Design review of the part built by this model. Coordinates are the model's own, in mm. A direction names the side the tool comes from. Round coordinates to 2 decimals unless told otherwise and drop trailing zeros. Order: outer loops, then holes, each group sorted by start corner. A loop starts at its lowest first (then second) coordinate and runs counter-clockwise, first axis right, second up.
from build123d import *

# Parameters (mm, degrees)
CUT_EXTRUDE_2_REACH      = 9.602
PATTERN_CIRCULAR_3_COUNT = 11
SKETCH_7_R               = 3.7
EXTRUDE_1_DEPTH          = 0.5
SKETCH_8_R               = 1.75
CUT_EXTRUDE_3_DEPTH      = 0.25
EXTRUDE_START            = 0.5
SKETCH_9_R               = 3.7
EXTRUDE_2_DEPTH          = 0.5
SKETCH_11_R              = 1.55
CUT_EXTRUDE_5_DEPTH      = 3
SKETCH_13_R              = 0.5625
CUT_EXTRUDE_7_DEPTH      = 9.739565207


with BuildPart() as part:
    # Sketch 1 → Revolve 1 (revolve)
    with BuildSketch(Plane.XY, mode=Mode.PRIVATE) as revolve_1_sk:
        Polygon((0, 1), (0, 3.301), (6, 3.301), (6, 2.2264), (6, 1), align=None)
    revolve(revolve_1_sk.sketch.rotate(Axis((0, 0, 0), (1, 0, 0)), 90), axis=Axis((0, 0, 0), (1, 0, 0)))

    # Sketch 6 → Cut-Extrude 2 (cut, up to next)
    with BuildSketch(Plane(origin=(0, 0, 0), x_dir=(0, 0, -1), z_dir=(1, 0, 0)), mode=Mode.PRIVATE) as cut_extrude_2_sk1:
        with BuildLine():
            Line((0.620299767, 3.127317535), (0.514085384, 2.835495915))
            ThreePointArc((0.514085384, 2.835495915), (0.376876254, 2.662359121), (0.163302545, 2.605888194))
            ThreePointArc((0.163302545, 2.605888194), (0, 2.611), (-0.163302545, 2.605888194))
            ThreePointArc((-0.163302545, 2.605888194), (-0.376876254, 2.662359121), (-0.514085384, 2.835495915))
            Line((-0.514085384, 2.835495915), (-0.620299767, 3.127317535))
            ThreePointArc((-0.620299767, 3.127317535), (-0.680969197, 3.197392704), (-0.772898084, 3.209241273))
            ThreePointArc((-0.772898084, 3.209241273), (-0.835941408, 3.193399906), (-0.898660577, 3.176320224))
            Line((-0.898660577, 3.176320224), (-1.396756451, 4.544827391))
            ThreePointArc((-1.396756451, 4.544827391), (0, 4.754617188), (1.396756451, 4.544827391))
            Line((1.396756451, 4.544827391), (0.898660577, 3.176320224))
            ThreePointArc((0.898660577, 3.176320224), (0.835941408, 3.193399906), (0.772898084, 3.209241273))
            ThreePointArc((0.772898084, 3.209241273), (0.680969197, 3.197392704), (0.620299767, 3.127317535))
        make_face()
    cut_extrude_2_tool1 = extrude(cut_extrude_2_sk1.sketch, amount=CUT_EXTRUDE_2_REACH, mode=Mode.PRIVATE) & part.part
    cut_extrude_2 = cut_extrude_2_tool1.solids().sort_by_distance((0, 3.839085, 0))[0]
    add(cut_extrude_2, mode=Mode.SUBTRACT)

    # Pattern Circular 3: Cut-Extrude 2 ×11 about axis
    pattern_circular_3_axis = Axis((0, 0, 0), (1, 0, 0))
    for i in range(1, PATTERN_CIRCULAR_3_COUNT):
        add(cut_extrude_2.rotate(pattern_circular_3_axis, i * 360 / PATTERN_CIRCULAR_3_COUNT), mode=Mode.SUBTRACT)

    # Sketch 7 → Extrude 1 (add)
    with BuildSketch(Plane.ZY):
        Circle(SKETCH_7_R)
    extrude(amount=EXTRUDE_1_DEPTH)

    # Sketch 8 → Cut-Extrude 3 (cut)
    with BuildSketch(Plane.ZY.offset(0.5)):
        Circle(SKETCH_8_R)
    extrude(amount=-CUT_EXTRUDE_3_DEPTH, mode=Mode.SUBTRACT)

    # Sketch 9 → Extrude 2 (add)
    with BuildSketch(Plane(origin=(6, 0, 0), x_dir=(0, 0, -1), z_dir=(1, 0, 0)).offset(EXTRUDE_START)):
        with Locations(Location((0, 0, 0), (0, 0, 180))):
            Circle(SKETCH_9_R)
    extrude(amount=-EXTRUDE_2_DEPTH)

    # Sketch 11 → Cut-Extrude 5 (cut)
    with BuildSketch(Plane.ZY.offset(0.25)):
        Circle(SKETCH_11_R)
    extrude(amount=-CUT_EXTRUDE_5_DEPTH, mode=Mode.SUBTRACT)

    # Sketch 13 → Cut-Extrude 7 (cut, through all)
    with BuildSketch(Plane(origin=(6.5, 0, 0), x_dir=(0, 0, -1), z_dir=(1, 0, 0))):
        Circle(SKETCH_13_R)
    extrude(amount=-CUT_EXTRUDE_7_DEPTH, mode=Mode.SUBTRACT)


solid = part.part
1) Take a section at A-A on z = 0. Give the boundary of the cut face in (x, y), plus the area to 3 significant figures.
Results:
outline: (-0.5, -3.7) - (0, -3.7) - (0, -3.3) - (6, -3.3) - (6, -3.7) - (6.5, -3.7) - (6.5, -0.56) - (6, -0.56) - (6, -1) - (2.75, -1) - (2.75, -1.55) - (-0.25, -1.55) - (-0.25, -1.75) - (-0.5, -1.75) - close; (-0.5, 1.75) - (-0.25, 1.75) - (-0.25, 1.55) - (2.75, 1.55) - (2.75, 1) - (6, 1) - (6, 0.56) - (6.5, 0.56) - (6.5, 3.7) - (6, 3.7) - (6, 2.61) - (0, 2.61) - (0, 3.7) - (-0.5, 3.7) - close
area: 25.6 mm2
2) Take a section at B-B on y = 0. Give the boundary of the cut face in (x, z), plus the area to 3 significant figures.
Results:
outline: (-0.5, -3.7) - (0, -3.7) - (0, -2.69) - (6, -2.69) - (6, -3.7) - (6.5, -3.7) - (6.5, -0.56) - (6, -0.56) - (6, -1) - (2.75, -1) - (2.75, -1.55) - (-0.25, -1.55) - (-0.25, -1.75) - (-0.5, -1.75) - close; (-0.5, 1.75) - (-0.25, 1.75) - (-0.25, 1.55) - (2.75, 1.55) - (2.75, 1) - (6, 1) - (6, 0.56) - (6.5, 0.56) - (6.5, 3.7) - (6, 3.7) - (6, 2.69) - (0, 2.69) - (0, 3.7) - (-0.5, 3.7) - close
area: 22.5 mm2
3) Clearance check with flat-ended pins moving along their axes: P1, Ø1.5, axis at x = 5, y = -2, coming from the -Z side; P2, Ø3, axis at x = 1, y = -1.5, coming from the +Z side; P3, Ø0.6, axis at y = 0, z = 0, coming from the -X side; P4, Ø1, axis at y = 0.5, z = 0.5, coming from the -X side. State where each tip first meets the part, or that it passes through.
Results:
P1: stops at z = -3.06
P2: stops at z = 3.68
P3: passes through
P4: stops at x = 2.75
4) To check wall thickness, follow line 1 along X through (y, z) = (-1, 3); line 2 along Z through (x, y) = (4.5, 3); line 3 along X through (y, z) = (-0.75, 1.5). State the ranges of each line that lie inside material, in increasing order.
Results:
line 1: x = -0.5 to 0, 6 to 6.5
line 2: z = -1.17 to -0.57, 0.57 to 1.17
line 3: x = -0.25 to 6.5
5) For faces 1 (the face through (-0.246, -3.612, -0.802)), 2 (the face through (1.229, -1.375, 0.715)), 3 (the face through (6, -2, 2)), list the 3-axis set-ups (+Z, -Z, +X, -X, +Y, -Y) from which the entire face can be reached by the end or side of a thin tool; tool diameter is ignored.
Results:
face 1: +X, -X
face 2: -X
face 3: none
6) The part is to be moulded in two halves that separate along X. For faces 4 (the face through (-0.5, -2, 1)), 5 (the face through (4, 1, 0)), 6 (the face through (0, -2, -2)), say which applies: released by +X, released by -X, zero draft, split by the parting line, or undercut.
Results:
face 4: released by -X
face 5: zero draft
face 6: undercut
